Here's how the part is built. I have some questions about the finished solid (model axes, mm). A direction names the side the tool comes from. Give positions to 0.01 mm unless a question says otherwise; leave off trailing zeros. Write each loop counter-clockwise with the first axis right and the second up, starting at its lowest first coordinate (ties: lowest second). Pieces come first, ordered by that corner, then holes. Notation, with made-up numbers: (80.25, -5.5) - (95.25, -5.5) arc R27 cw to (95.25, 16.5) - close; hole circle Ø1 at (77.5, 56.25). An arc over 180 degrees is marked (long way). Use a Markdown table: item, result.
```python
from build123d import *

# Parameters (mm, degrees)
SKETCH1_W           = 46
SKETCH1_H           = 32
SKETCH1_R           = 7
BOSS_EXTRUDE1_DEPTH = 22.5
SKETCH2_R           = 11
CUT_EXTRUDE1_DEPTH  = 8
CUT_EXTRUDE2_START  = -8
SKETCH3_R           = 11
CUT_EXTRUDE2_DEPTH  = 8
SKETCH4_R           = 1.65
CUT_EXTRUDE3_DEPTH  = 10
CHAMFER1_SIZE       = 0.5
SKETCH5_W           = 46
SKETCH5_H           = 45
BOSS_EXTRUDE2_DEPTH = 6
SKETCH6_R           = 1.65
CUT_EXTRUDE4_DEPTH  = 8
SKETCH8_W           = 46
SKETCH8_H           = 45
BOSS_EXTRUDE3_DEPTH = 5


with BuildPart() as part:
    # Sketch1 → Boss-Extrude1 (new, symmetric)
    with BuildSketch(Plane.XY):
        Rectangle(SKETCH1_W, SKETCH1_H)
        with Locations(Location((0, 0, 0), (0, 0, 180))):
            Circle(SKETCH1_R, mode=Mode.SUBTRACT)
    extrude(amount=BOSS_EXTRUDE1_DEPTH, both=True)

    # Sketch2 → Cut-Extrude1 (cut)
    with BuildSketch(Plane.XY.offset(22.5)):
        Circle(SKETCH2_R)
    extrude(amount=-CUT_EXTRUDE1_DEPTH, mode=Mode.SUBTRACT)

    # Sketch3 → Cut-Extrude2 (cut)
    with BuildSketch(Plane(origin=(0, 0, -22.5), x_dir=(-1, 0, 0), z_dir=(0, 0, -1)).offset(CUT_EXTRUDE2_START)):
        with Locations(Location((0, 0, 0), (0, 0, 180))):
            Circle(SKETCH3_R)
    extrude(amount=CUT_EXTRUDE2_DEPTH, mode=Mode.SUBTRACT)

    # Sketch4 → Cut-Extrude3 (cut)
    with BuildSketch(Plane.ZY.offset(23)):
        with Locations((12, -9)):
            Circle(SKETCH4_R)
        with Locations((12, 9)):
            Circle(SKETCH4_R)
        with Locations((-12, -9)):
            Circle(SKETCH4_R)
        with Locations((-12, 9)):
            Circle(SKETCH4_R)
    cut_extrude3 = extrude(amount=-CUT_EXTRUDE3_DEPTH, mode=Mode.SUBTRACT)

    # Mirror1: Cut-Extrude3 across plane
    add(cut_extrude3.mirror(Plane(origin=(0, 0, 0), x_dir=(0, 0, 1), z_dir=(1, 0, 0))), mode=Mode.SUBTRACT)

    # Chamfer1
    chamfer1_edges = [part.edges().sort_by_distance(p)[0] for p in [
        (7, 0, 14.5),
        (-11, 0, 22.5),
        (7, 0, -14.5),
        (-11, 0, -22.5),
    ]]
    chamfer(chamfer1_edges, length=CHAMFER1_SIZE)

    # Sketch5 → Boss-Extrude2 (add)
    with BuildSketch(Plane(origin=(0, 16, 0), x_dir=(1, 0, 0), z_dir=(0, 1, 0))):
        Rectangle(SKETCH5_W, SKETCH5_H)
        with BuildLine():
            Line((-10, -15.25), (-15, -15.25))
            ThreePointArc((-15, -15.25), (-16.75, -13.5), (-15, -11.75))
            Line((-15, -11.75), (-10, -11.75))
            ThreePointArc((-10, -11.75), (-8.25, -13.5), (-10, -15.25))
        make_face(mode=Mode.SUBTRACT)
        with BuildLine():
            Line((10, 16.25), (15, 16.25))
            ThreePointArc((15, 16.25), (16.75, 14.5), (15, 12.75))
            Line((15, 12.75), (10, 12.75))
            ThreePointArc((10, 12.75), (8.25, 14.5), (10, 16.25))
        make_face(mode=Mode.SUBTRACT)
        with BuildLine():
            Line((15, -11.75), (10, -11.75))
            ThreePointArc((10, -11.75), (8.25, -13.5), (10, -15.25))
            Line((10, -15.25), (15, -15.25))
            ThreePointArc((15, -15.25), (16.75, -13.5), (15, -11.75))
        make_face(mode=Mode.SUBTRACT)
        with BuildLine():
            Line((-15, 12.75), (-10, 12.75))
            ThreePointArc((-10, 12.75), (-8.25, 14.5), (-10, 16.25))
            Line((-10, 16.25), (-15, 16.25))
            ThreePointArc((-15, 16.25), (-16.75, 14.5), (-15, 12.75))
        make_face(mode=Mode.SUBTRACT)
    extrude(amount=BOSS_EXTRUDE2_DEPTH)

    # Sketch6 → Cut-Extrude4 (cut)
    with BuildSketch(Plane(origin=(0, 0, -22.5), x_dir=(-1, 0, 0), z_dir=(0, 0, -1))):
        with Locations((15, 0)):
            Circle(SKETCH6_R)
        with Locations((-15, 0)):
            Circle(SKETCH6_R)
    cut_extrude4 = extrude(amount=-CUT_EXTRUDE4_DEPTH, mode=Mode.SUBTRACT)

    # Mirror2: Cut-Extrude4 across plane
    add(cut_extrude4.mirror(Plane.XY), mode=Mode.SUBTRACT)

    # Sketch8 → Boss-Extrude3 (add)
    with BuildSketch(Plane.XZ.offset(16)):
        Rectangle(SKETCH8_W, SKETCH8_H)
    extrude(amount=BOSS_EXTRUDE3_DEPTH)


solid = part.part
```
Item 1: If we section it at B-B, the plane x = 0: Write out the boundary of the cut face in (y, z).
Values:
| item | result |
|---|---|
| outline | (-21, -22.5) - (-11.5, -22.5) - (-11, -22) - (-11, -14.5) - (-7.5, -14.5) - (-7, -14) - (-7, 14) - (-7.5, 14.5) - (-11, 14.5) - (-11, 22) - (-11.5, 22.5) - (-21, 22.5) - close; (7, -14) - (7.5, -14.5) - (11, -14.5) - (11, -22) - (11.5, -22.5) - (22, -22.5) - (22, 22.5) - (11.5, 22.5) - (11, 22) - (11, 14.5) - (7.5, 14.5) - (7, 14) - close |
Item 2: If we section it at A-A, the plane z = -12: Write out the boundary of the cut face in (x, y).
Values:
| item | result |
|---|---|
| outline | (-23, -21) - (23, -21) - (23, -10.65) - (13, -10.65) - (13, -7.35) - (23, -7.35) - (23, 7.35) - (13, 7.35) - (13, 10.65) - (23, 10.65) - (23, 22) - (-23, 22) - (-23, 10.65) - (-13, 10.65) - (-13, 7.35) - (-23, 7.35) - (-23, -7.35) - (-13, -7.35) - (-13, -10.65) - (-23, -10.65) - close; hole circle Ø14 at (0, 0) |
Item 3: Will these pins go through, and if not, where does the flat tip stop? pin 1 Ø1 at (y, z) = (9, -11.5) entering from -X; pin 2 Ø1 at (y, z) = (9, -11.5) entering from +X; pin 3 Ø1.6 at (x, y) = (15, 0.5) entering from -Z.
Values:
| item | result |
|---|---|
| pin 1 | stops at x = -13 |
| pin 2 | stops at x = 13 |
| pin 3 | stops at z = -14.5 |
Item 4: If we section it at C-C, the plane z = -17: Write out the boundary of the cut face in (x, y), plus the area to 3 significant figures.
Values:
| item | result |
|---|---|
| outline | (-23, -21) - (23, -21) - (23, 22) - (-23, 22) - close; hole circle Ø3.3 at (-15, 0); hole circle Ø22 at (0, 0); hole circle Ø3.3 at (15, 0) |
| area | 1,580 mm2 |
Item 5: If we section it at D-D, the plane z = 4.5: Write out the boundary of the cut face in (x, y), plus the area to 3 significant figures.
Values:
| item | result |
|---|---|
| outline | (-23, -21) - (23, -21) - (23, 22) - (-23, 22) - close; hole circle Ø14 at (0, 0) |
| area | 1,820 mm2 |
Item 6: Thinking about a two-plate mould opening in X: for faces 1 (the flat face through (15, 0, -14.5)), 2 (the flat face through (13, -9, -12)), 3 (the cylindrical face through (-18.07, 8.368, 13.524)), 4 (the flat face through (-23, 1, 0)), which applies, +X half, -X half, draft (parallel to the pull), parting line (faces both ways), or undercut?
Values:
| item | result |
|---|---|
| face 1 | undercut |
| face 2 | +X half |
| face 3 | draft |
| face 4 | -X half |
Item 7: For faces 5 (the flat face through (13, 9, -12)), 6 (the flat face through (15, 0, 14.5)), 7 (the flat face through (12, 19, -16.25)), which set-ups out of +Z, -Z, +X, -X, +Y, -Y let a thin tool reach every point of the face, with its end or its side?
Values:
| item | result |
|---|---|
| face 5 | +X |
| face 6 | +Z |
| face 7 | +Y |
Item 8: I need wall thicknesses on line 1 along Y through (x, z) = (-17.75, -12); line 2 along Y through (x, z) = (0, -2); line 3 along Y through (x, z) = (14, -10.5). Which ranges of each line are inside material? Lowest first, please. Write a range as [from, to].
Values:
| item | result |
|---|---|
| line 1 | y = [-21, -10.65], [-7.35, 7.35], [10.65, 22] |
| line 2 | y = [-21, -7], [7, 22] |
| line 3 | y = [-21, -9.69], [-8.31, 8.31], [9.69, 22] |
